```python
from build123d import *

# Parameters (mm, degrees)
SKETCH1_R           = 42.5
BOSS_EXTRUDE1_DEPTH = 2.5
SKETCH3_W           = 13
SKETCH3_H           = 18
BOSS_EXTRUDE2_DEPTH = 20
SKETCH4_R           = 8.5
CUT_EXTRUDE2_DEPTH  = 20
SKETCH5_R           = 8.5
CUT_EXTRUDE3_DEPTH  = 20
SKETCH6_R           = 8.5
CUT_EXTRUDE4_DEPTH  = 20
CUT_EXTRUDE5_START  = -20
SKETCH7_R           = 8.5
CUT_EXTRUDE5_DEPTH  = 20
CUT_EXTRUDE6_START  = -20
SKETCH8_R           = 8.5
CUT_EXTRUDE6_DEPTH  = 20
CUT_EXTRUDE7_START  = -20
SKETCH9_R           = 8.5
CUT_EXTRUDE7_DEPTH  = 20
CUT_EXTRUDE8_DEPTH  = 76.388
SKETCH11_W          = 71.811217628
SKETCH11_H          = 11.984599711
CUT_EXTRUDE9_DEPTH  = 76.388
SKETCH12_R          = 18.204170311
CUT_EXTRUDE10_DEPTH = 76.388
SKETCH13_R          = 1.997627935
CUT_EXTRUDE11_DEPTH = 10
CUT_EXTRUDE13_START = -24
SKETCH15_R          = 42.5
SKETCH15_R_2        = 34
CUT_EXTRUDE13_DEPTH = 24


with BuildPart() as part:
    # Sketch1 → Boss-Extrude1 (new body)
    with BuildSketch(Plane(origin=(0, 0, 0), x_dir=(1, 0, 0), z_dir=(0, 1, 0))):
        with Locations(Location((0, 0, 0), (0, 0, 270))):
            Circle(SKETCH1_R)
    extrude(amount=BOSS_EXTRUDE1_DEPTH)

    # Sketch3 → Boss-Extrude2 (add)
    with BuildSketch(Plane(origin=(0, 2.5, 0), x_dir=(1, 0, 0), z_dir=(0, 1, 0))):
        with Locations((-26.394376419, 0)):
            Rectangle(SKETCH3_W, SKETCH3_H)
        with Locations((26.394376419, 0)):
            Rectangle(SKETCH3_W, SKETCH3_H)
        Polygon((-8.599367677, 32.894541729), (-2.099367677, 21.63621148), (-17.687824945, 12.63621148), (-24.187824945, 23.894541729), align=None)
        Polygon((8.599367677, 32.894541729), (24.187824945, 23.894541729), (17.687824945, 12.63621148), (2.099367677, 21.63621148), align=None)
        Polygon((8.599367677, -32.894541729), (2.099367677, -21.63621148), (17.687824945, -12.63621148), (24.187824945, -23.894541729), align=None)
        Polygon((-8.599367677, -32.894541729), (-24.187824945, -23.894541729), (-17.687824945, -12.63621148), (-2.099367677, -21.63621148), align=None)
    extrude(amount=BOSS_EXTRUDE2_DEPTH)

    # Sketch4 → Cut-Extrude2 (cut)
    with BuildSketch(Plane.ZY.offset(32.894376419)):
        with Locations((0, 12.5)):
            Circle(SKETCH4_R)
    extrude(amount=-CUT_EXTRUDE2_DEPTH, mode=Mode.SUBTRACT)

    # Sketch5 → Cut-Extrude3 (cut)
    with BuildSketch(Plane(origin=(-16.393596311, 0, 28.394541729), x_dir=(0.8660254037844386, 0, 0.5000000000000003), z_dir=(-0.5000000000000003, 0, 0.8660254037844386))):
        with Locations((0, 12.5)):
            Circle(SKETCH5_R)
    extrude(amount=-CUT_EXTRUDE3_DEPTH, mode=Mode.SUBTRACT)

    # Sketch6 → Cut-Extrude4 (cut)
    with BuildSketch(Plane(origin=(16.393596311, 0, 28.394541729), x_dir=(0.8660254037844386, 0, -0.5000000000000003), z_dir=(0.5000000000000003, 0, 0.8660254037844386))):
        with Locations((0, 12.5)):
            Circle(SKETCH6_R)
    extrude(amount=-CUT_EXTRUDE4_DEPTH, mode=Mode.SUBTRACT)

    # Sketch7 → Cut-Extrude5 (cut)
    with BuildSketch(Plane(origin=(32.894376419, 0, 0), x_dir=(0, 0, -1), z_dir=(1, 0, 0)).offset(CUT_EXTRUDE5_START)):
        with Locations(Location((0, 12.5, 0), (0, 0, 180))):
            Circle(SKETCH7_R)
    extrude(amount=CUT_EXTRUDE5_DEPTH, mode=Mode.SUBTRACT)

    # Sketch8 → Cut-Extrude6 (cut)
    with BuildSketch(Plane(origin=(16.393596311, 0, -28.394541729), x_dir=(-0.8660254037844386, 0, -0.5000000000000003), z_dir=(0.5000000000000003, 0, -0.8660254037844386)).offset(CUT_EXTRUDE6_START)):
        with Locations(Location((0, 12.5, 0), (0, 0, 180))):
            Circle(SKETCH8_R)
    extrude(amount=CUT_EXTRUDE6_DEPTH, mode=Mode.SUBTRACT)

    # Sketch9 → Cut-Extrude7 (cut)
    with BuildSketch(Plane(origin=(-16.393596311, 0, -28.394541729), x_dir=(-0.8660254037844386, 0, 0.5000000000000003), z_dir=(-0.5000000000000003, 0, -0.8660254037844386)).offset(CUT_EXTRUDE7_START)):
        with Locations(Location((0, 12.5, 0), (0, 0, 180))):
            Circle(SKETCH9_R)
    extrude(amount=CUT_EXTRUDE7_DEPTH, mode=Mode.SUBTRACT)

    # Sketch10 → Cut-Extrude8 (cut)
    with BuildSketch(Plane(origin=(-16.393596311, 0, -28.394541729), x_dir=(-0.8660254037844386, 0, 0.5000000000000003), z_dir=(-0.5000000000000003, 0, -0.8660254037844386))):
        Polygon((-35.669118209, 17.957805899), (-9, 17.957805899), (-9, 22.5), (-6.516314508, 22.5), (-6.516314508, 25.559573076), (-35.669118209, 25.559573076), align=None)
        Polygon((-6.516314508, 25.559573076), (-6.516314508, 22.5), (9, 22.5), (9, 17.957805899), (33.747549551, 17.957805899), (33.747549551, 25.559573076), align=None)
    extrude(amount=-CUT_EXTRUDE8_DEPTH, mode=Mode.SUBTRACT)

    # Sketch11 → Cut-Extrude9 (cut)
    with BuildSketch(Plane(origin=(-16.393596311, 0, -28.394541729), x_dir=(-0.8660254037844386, 0, 0.5000000000000003), z_dir=(-0.5000000000000003, 0, -0.8660254037844386))):
        with Locations((1.515702587, 16.507700144)):
            Rectangle(SKETCH11_W, SKETCH11_H)
    extrude(amount=-CUT_EXTRUDE9_DEPTH, mode=Mode.SUBTRACT)

    # Sketch12 → Cut-Extrude10 (cut)
    with BuildSketch(Plane(origin=(0, 2.5, 0), x_dir=(1, 0, 0), z_dir=(0, 1, 0))):
        with Locations(Location((0, 0, 0), (0, 0, 270))):
            Circle(SKETCH12_R)
    extrude(amount=-CUT_EXTRUDE10_DEPTH, mode=Mode.SUBTRACT)

    # Sketch13 → Cut-Extrude11 (cut)
    with BuildSketch(Plane(origin=(0, 2.5, 0), x_dir=(1, 0, 0), z_dir=(0, 1, 0))):
        with Locations(Location((-22.072556502, 12.515367089, 0), (0, 0, 270))):
            Circle(SKETCH13_R)
        with Locations(Location((22.072556502, 12.515367089, 0), (0, 0, 270))):
            Circle(SKETCH13_R)
        with Locations(Location((22.072556502, -12.515367089, 0), (0, 0, 270))):
            Circle(SKETCH13_R)
        with Locations(Location((-22.072556502, -12.515367089, 0), (0, 0, 270))):
            Circle(SKETCH13_R)
    extrude(amount=-CUT_EXTRUDE11_DEPTH, mode=Mode.SUBTRACT)

    # Sketch15 → Cut-Extrude13 (cut)
    with BuildSketch(Plane(origin=(0, 2.5, 0), x_dir=(1, 0, 0), z_dir=(0, 1, 0)).offset(CUT_EXTRUDE13_START)):
        Circle(SKETCH15_R)
        with Locations(Location((0, 0, 0), (0, 0, 270))):
            Circle(SKETCH15_R_2, mode=Mode.SUBTRACT)
    extrude(amount=CUT_EXTRUDE13_DEPTH, mode=Mode.SUBTRACT)


solid = part.part
```
The model under review builds one solid part; all positions refer to its coordinate system, in mm. A direction names the side the tool comes from. Give positions to 0.01 mm unless a question says otherwise; leave off trailing zeros. Loops run counter-clockwise (first coordinate to the right, second up) from the corner with the lowest first, then second, coordinate; pieces in that order, holes last. Notation, with made-up numbers: (-27.5, 45) - (3.5, 45) arc R28 cw to (3.5, 65) - close; hole circle Ø8 at (51, 8.25). An arc over 180 degrees is marked (long way). Answer as a JSON object with one key per item and string values.
Q1. For faces 4 (the flat face through (-20.98, 6.45, 18.34)), 5 (the flat face through (19.6, 2.5, -0.2)), 6 (the flat face through (16, 2.5, -29)), list the 3-axis set-ups (+Z, -Z, +X, -X, +Y, -Y) from which the entire face can be reached by the end or side of a thin tool; tool diameter is ignored.
Worked out:
{"face 4": "-X, +Y", "face 5": "+Y", "face 6": "-Z, +X, +Y"}
Q2. Insertion check: pin 1 (6 mm diameter, centred on x = 14.5, y = 1.5, fed in from +Z); pin 2 (4 mm diameter, centred on y = 5, z = 2.5, fed in from -X); pin 3 (2 mm diameter, centred on y = 4, z = -6.5, fed in from +X); pin 4 (8 mm diameter, centred on x = -8.5, z = 10.5, fed in from +Y). Each pin has a flat end and moves straight along its axis. Give the tip position at first contact, or say it passes through.
Worked out:
{"pin 1": "stops at z = 32", "pin 2": "stops at x = -32.89", "pin 3": "stops at x = 32.89", "pin 4": "passes through"}
Q3. Add section B-B on x = 0. State the section outline as (y, z) points, plus the area to 3 significant figures.
Worked out:
{"outline": "(0, -34) - (2.5, -34) - (2.5, -18.2) - (0, -18.2) - close; (0, 18.2) - (2.5, 18.2) - (2.5, 34) - (0, 34) - close", "area": "79.0 mm^2"}
Q4. Mouldability with a two-part tool opening along Z and no side actions: class faces 1 (the flat face through (9.78, 3.78, 17.2)), 2 (the flat face through (-16.28, 3.78, 28.46)), 3 (the cylindrical face through (33.71, 1.23, -4.43)) as +Z half, -Z half, draft (parallel to the pull), parting line (faces both ways), or undercut.
Worked out:
{"face 1": "undercut", "face 2": "+Z half", "face 3": "parting line"}
Q5. Add section C-C on x = 30. State the section outline as (y, z) points, plus the area to 3 significant figures.
Worked out:
{"outline": "(0, -16) - (2.5, -16) - (2.5, -9) - (10.52, -9) - (10.52, -8.27) arc R8.5 cw to (10.52, 8.27) - (10.52, 9) - (2.5, 9) - (2.5, 16) - (0, 16) - close", "area": "144 mm^2"}
Q6. Add section A-A on z = 0. State the section outline as (x, y) points, plus the area to 3 significant figures.
Worked out:
{"outline": "(-34, 0) - (-18.2, 0) - (-18.2, 2.5) - (-19.89, 2.5) - (-19.89, 4) - (-32.89, 4) - (-32.89, 2.5) - (-34, 2.5) - close; (18.2, 0) - (34, 0) - (34, 2.5) - (32.89, 2.5) - (32.89, 4) - (19.89, 4) - (19.89, 2.5) - (18.2, 2.5) - close", "area": "118 mm^2"}
Q7. Add section D-D on y = 1.5. State the section outline as (x, z) points.
Worked out:
{"outline": "circle Ø68 at (0, 0); hole circle Ø4 at (-22.07, -12.52); hole circle Ø4 at (-22.07, 12.52); hole circle Ø36.41 at (0, 0); hole circle Ø4 at (22.07, -12.52); hole circle Ø4 at (22.07, 12.52)"}
Q8. To check wall thickness, follow line 1 along X through (y, z) = (3, -6.5); line 2 along Y through (x, z) = (13.5, -14.5); line 3 along Z through (x, y) = (-2.5, 7.75). State the ranges of each line that lie inside material, in increasing order.
Worked out:
{"line 1": "x = -32.89 to -19.89, 19.89 to 32.89", "line 2": "y = 0 to 2.5", "line 3": "z = -22.33 to -21.4, 21.4 to 22.33"}
